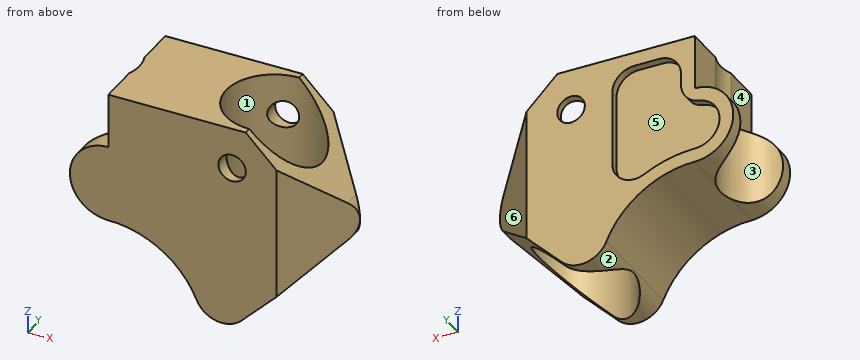
from build123d import *

# Parameters (mm, degrees)
BOSS_EXTRU_1_DEPTH      = 20
ENL_V_MAT_EXTRU_1_DEPTH = 3
ESQUISSE3_R             = 17.5
ESQUISSE3_R_2           = 15
ENL_V_MAT_EXTRU_2_DEPTH = 113.493063486
ESQUISSE5_R             = 5
ENL_V_MAT_EXTRU_3_DEPTH = 118.705944436
ENL_V_MAT_EXTRU_4_DEPTH = 113.493063571


with BuildPart() as part:
    # Esquisse1 → Boss.-Extru.1 (new, symmetric)
    with BuildSketch(Plane(origin=(0, 0, 0), x_dir=(1, 0, 0), z_dir=(0, 1, 0))):
        with BuildLine():
            Line((0, 0), (50, 0))
            Line((50, 0), (78.284271247, 28.284271247))
            ThreePointArc((78.284271247, 28.284271247), (81.213203436, 35.355339059), (78.284271247, 42.426406871))
            Line((78.284271247, 42.426406871), (48.412587767, 72.298090352))
            ThreePointArc((48.412587767, 72.298090352), (39.455979063, 75.047650602), (32.154515521, 69.176573087))
            ThreePointArc((32.154515521, 69.176573087), (19.250715026, 53.76970799), (0, 48))
            ThreePointArc((0, 48), (-14, 34), (0, 20))
            Line((0, 20), (0, 0))
        make_face()
    extrude(amount=BOSS_EXTRU_1_DEPTH, both=True)

    # Esquisse2 → Enlèv. mat.-Extru.1 (cut)
    with BuildSketch(Plane(origin=(0, 20, 0), x_dir=(1, 0, 0), z_dir=(0, 1, 0))):
        with BuildLine():
            Line((30, 40.338541985), (30, 13))
            ThreePointArc((30, 13), (27.656854249, 7.343145751), (22, 5))
            Line((22, 5), (13, 5))
            ThreePointArc((13, 5), (7.343145751, 7.343145751), (5, 13))
            Line((5, 13), (5, 17.266799469))
            ThreePointArc((5, 17.266799469), (3.135719911, 22.400311053), (-1.588235294, 25.141246778))
            ThreePointArc((-1.588235294, 25.141246778), (-8.964618759, 34.797251843), (0, 43))
            ThreePointArc((0, 43), (9.432693133, 44.128103979), (18.333333333, 47.448784987))
            ThreePointArc((18.333333333, 47.448784987), (26.163331999, 47.169842495), (30, 40.338541985))
        make_face()
    extrude(amount=-ENL_V_MAT_EXTRU_1_DEPTH, mode=Mode.SUBTRACT)

    # Esquisse3 → Enlèv. mat.-Extru.2 (cut, through all)
    with BuildSketch(Plane.XY):
        with Locations(Location((50, 0, 0), (0, 0, 270))):
            Circle(ESQUISSE3_R)
        with Locations((-14, 0)):
            Circle(ESQUISSE3_R_2)
    extrude(amount=-ENL_V_MAT_EXTRU_2_DEPTH, mode=Mode.SUBTRACT)

    # Esquisse5 → Enlèv. mat.-Extru.3 (cut, through all)
    with BuildSketch(Plane(origin=(0, 20, 0), x_dir=(1, 0, 0), z_dir=(0, 1, 0))):
        with Locations(Location((45, 15, 0), (0, 0, 270))):
            Circle(ESQUISSE5_R)
    extrude(amount=-ENL_V_MAT_EXTRU_3_DEPTH, mode=Mode.SUBTRACT)

    # Esquisse6 → Enlèv. mat.-Extru.4 (cut, through all)
    with BuildSketch(Plane.XY):
        Polygon((81.213203436, 0), (81.213203436, 20), (61.213203436, 20), align=None)
        Polygon((81.213203436, -20), (81.213203436, 0), (61.213203436, -20), align=None)
    extrude(amount=-ENL_V_MAT_EXTRU_4_DEPTH, mode=Mode.SUBTRACT)


solid = part.part
Design review of the part built by this model. Coordinates are the model's own, in mm. Face numbers are marked on the shaded views. A direction names the side the tool comes from. Give positions to 0.01 mm unless a question says otherwise; leave off trailing zeros. Loops run counter-clockwise (first coordinate to the right, second up) from the corner with the lowest first, then second, coordinate; pieces in that order, holes last. Notation, with made-up numbers: M 39,-4.5 L 93,-4.5 A23 cw 93,8.5 Z; hole C 2.25,-23.75 d6. An arc over 180 degrees is marked long. Write item = value, one per line.
Q1. We need section D-D (y = -9). Give the boundary of the cut face in (x, z), plus the area to 3 significant figures.
Output values:
outline = M -2,-47.86 A14 ccw 0,-48 A35 cw 32.15,-69.18 A10 ccw 34.99,-72.95 L 34.99,0 L 0,0 L 0,-20 A14 ccw -2,-20.14 Z; M 65.01,-55.7 L 72.21,-48.5 L 72.21,-22.21 L 65.01,-15.01 Z
area = 2,230 mm^2
Q2. We need section B-B (z = -15). Give the boundary of the cut face in (x, y).
Output values:
outline = M 0,-20 L 40,-20 L 40,-14.36 A17.5 cw 40,14.36 L 40,20 L 30,20 L 30,17 L 5,17 L 5,20 L 0,20 L 0,5.39 A15 cw 0,-5.39 Z; M 50,-20 L 61.21,-20 L 65,-16.21 L 65,-9.01 A17.5 cw 50,-17.5 Z; M 50,17.5 A17.5 cw 65,9.01 L 65,16.21 L 61.21,20 L 50,20 Z
Q3. Insertion check: pin 1 (11.5 mm diameter, centred on y = -15, z = -14, fed in from -X); pin 2 (10 mm diameter, centred on x = 17, y = 7.5, fed in from +Z); pin 3 (3 mm diameter, centred on y = -2.5, z = -24.5, fed in from -X); pin 4 (6 mm diameter, centred on y = -10, z = -21.5, fed in from +X). Each pin has a flat end and moves straight along its axis. Give the tip position at first contact, or say it passes through.
Output values:
pin_1 = 0
pin_2 = 0
pin_3 = 0.46
pin_4 = 73.47
Q4. To check wall thickness, follow line 1 (Z direction, x = 1, y = 12); line 2 (Y direction, x = 65, z = -34.5); line 3 (Z direction, x = 45, y = 18.5). State the ranges of each line that lie inside material, in increasing order. Write a range as [from, to].
Output values:
line_1 = [-48.01, 0]
line_2 = [-16.21, -9.01], [9.01, 16.21]
line_3 = [-74.53, -20], [-10, 0]
Q5. We need section A-A (x = 47). Give the boundary of the cut face in (y, z).
Output values:
outline = M -20,-73.47 L -17.24,-73.47 L -17.24,-19.58 L -20,-19.58 Z; M -20,-10.42 L -17.24,-10.42 L -17.24,0 L -20,0 Z; M 17.24,-73.47 L 20,-73.47 L 20,-19.58 L 17.24,-19.58 Z; M 17.24,-10.42 L 20,-10.42 L 20,0 L 17.24,0 Z
Q6. Draft analysis for pull direction X (two halves, no side actions). For the marked faces 1, 2 and 3, state which applies: +X half, -X half, draft (parallel to the pull), parting line (faces both ways), or undercut.
Output values:
face_1 = undercut
face_2 = parting line
face_3 = -X half
Q7. We need section C-C (x = -5.5). Give the boundary of the cut face in (y, z), plus the area to 3 significant figures.
Output values:
outline = M -20,-46.87 L -12.36,-46.87 L -12.36,-21.13 L -20,-21.13 Z; M 12.36,-46.87 L 20,-46.87 L 20,-41.12 L 17,-41.12 L 17,-26.88 L 20,-26.88 L 20,-21.13 L 12.36,-21.13 Z
area = 351 mm^2
Q8. For the marked faces 4, 5 and 6, list the 3-axis set-ups (+Z, -Z, +X, -X, +Y, -Y) from which the entire face can be reached by the end or side of a thin tool; tool diameter is ignored.
Output values:
face_4 = +Z, -X, +Y, -Y
face_5 = +Y
face_6 = +Z, -Z, +X, +Y
